Can you work these out from the model? Positions are in its coordinate system, mm. A direction names the side the tool comes from. Coordinates: 2 decimals unless noted, no trailing zeros. Order: outer loops, then holes, each group sorted by start corner. A loop starts at its lowest first (then second) coordinate and runs counter-clockwise, first axis right, second up.
```python
from build123d import *

# Parameters (mm, degrees)
SKETCH1_W           = 30
SKETCH1_H           = 52
SKETCH1_R           = 1.9
BOSS_EXTRUDE1_DEPTH = 10
CHAMFER1_SIZE       = 15
CHAMFER1_SIZE2      = 2.644904711
SKETCH2_W           = 5
SKETCH2_H           = 7.355095289
SKETCH2_H_2         = 30
BOSS_EXTRUDE2_DEPTH = 10
SKETCH3_R           = 1
SKETCH3_R_2         = 1.5
SKETCH3_R_3         = 2
CUT_EXTRUDE1_DEPTH  = 35
CHAMFER2_SIZE       = 1


with BuildPart() as part:
    # Sketch1 → Boss-Extrude1 (new body)
    with BuildSketch(Plane.XY):
        with Locations((15, 6)):
            Rectangle(SKETCH1_W, SKETCH1_H)
        with Locations((4.5, 26.5)):
            Circle(SKETCH1_R, mode=Mode.SUBTRACT)
        with Locations((25.5, 26.5)):
            Circle(SKETCH1_R, mode=Mode.SUBTRACT)
        with Locations((25.5, 5.5)):
            Circle(SKETCH1_R, mode=Mode.SUBTRACT)
        with Locations((4.5, 5.5)):
            Circle(SKETCH1_R, mode=Mode.SUBTRACT)
    extrude(amount=BOSS_EXTRUDE1_DEPTH)

    # Chamfer1
    chamfer1_edges = [part.edges().sort_by_distance(p)[0] for p in [
        (15, -20, 0),
    ]]
    chamfer1_side = [part.faces().sort_by_distance(p)[0] for p in [
        (15, 5.700491631, 0),
    ]]
    chamfer(chamfer1_edges, length=CHAMFER1_SIZE, length2=CHAMFER1_SIZE2, reference=chamfer1_side[0])

    # Sketch2 → Boss-Extrude2 (add)
    with BuildSketch(Plane.XZ.offset(20)):
        Polygon((0, 10), (30, 10), (30, 50), (-55, 50), (-55, 20), (-55, 10), (-5, 10), align=None)
        Polygon((-5, 2.644904711), (-5, 10), (-55, 10), (-55, -30), (-5, -30), align=None)
        with Locations((-2.5, 6.322452356)):
            Rectangle(SKETCH2_W, SKETCH2_H)
        with Locations((-57.5, 35)):
            Rectangle(SKETCH2_W, SKETCH2_H_2)
    extrude(amount=-BOSS_EXTRUDE2_DEPTH)

    # Sketch3 → Cut-Extrude1 (cut)
    with BuildSketch(Plane(origin=(0, -10, 0), x_dir=(1, 0, 0), z_dir=(0, 1, 0))):
        with Locations(Location((-43.5, 8, 0), (0, 0, 270))):
            Circle(SKETCH3_R)
        with Locations(Location((-43.5, 3, 0), (0, 0, 270))):
            Circle(SKETCH3_R_2)
        with Locations(Location((-33.5, -33.25, 0), (0, 0, 270))):
            Circle(SKETCH3_R_3)
        with Locations(Location((-53.5, -33.25, 0), (0, 0, 270))):
            Circle(SKETCH3_R_3)
        with Locations(Location((-43.5, -33.25, 0), (0, 0, 270))):
            Circle(SKETCH3_R_3)
    extrude(amount=-CUT_EXTRUDE1_DEPTH, mode=Mode.SUBTRACT)

    # Chamfer2
    chamfer2_edges = [part.edges().sort_by_distance(p)[0] for p in [
        (0, 32, 5),
        (30, 32, 5),
        (-15, -10, 50),
        (30, -15, 50),
        (-30, -10, -30),
        (-5, -15, -30),
        (-55, -15, -30),
        (-55, -20, -5),
        (-15, -20, 50),
        (-30, -20, -30),
        (-55, -10, -5),
        (15, -10, 10),
        (0, -10, 6.322452355),
    ]]
    chamfer(chamfer2_edges, length=CHAMFER2_SIZE)


solid = part.part
```
1. Imagine slicing it at A-A on x = 4.5. Please give me the cut outline in (y, z), then the cut area to 3 significant figures.
Completed:
outline: (-20, 2.64) - (-5, 0) - (3.6, 0) - (3.6, 10) - (-9, 10) - (-10, 11) - (-10, 49) - (-11, 50) - (-19, 50) - (-20, 49) - close; (7.4, 0) - (24.6, 0) - (24.6, 10) - (7.4, 10) - close; (28.4, 0) - (32, 0) - (32, 10) - (28.4, 10) - close
area: 824 mm2
2. I'm going to push flat-ended pins straight in: pin 1 (5 mm diameter, centred on x = -28, z = -17, fed in from +Y); pin 2 (6.5 mm diameter, centred on x = -58, y = -15.5, fed in from -Z); pin 3 (12 mm diameter, centred on y = 4, z = 15.5, fed in from -X). Where does each tip first touch, or does it pass through?
Completed:
pin 1: stops at y = -10
pin 2: stops at z = -29.25
pin 3: stops at x = 0
3. On a 3-axis mill with a long thin cutter (end or side, diameter ignored), from which of +Z, -Z, +X, -X, +Y, -Y can I reach the whole of each face in a straight line? I mean faces 1 (the cylindrical face through (-35.274, -14.93, 34.173)), 2 (the flat face through (15, 12, 10)), 3 (the flat face through (-3, -15, 2.645)). Say none if no direction works.
Completed:
face 1: +Y, -Y
face 2: +Z, +X, -X, +Y
face 3: -Z, +Y, -Y
4. Imagine slicing it at C-C on x = -33.5. Please give me the cut outline in (y, z), then the cut area to 3 significant figures.
Completed:
outline: (-20, -29) - (-19, -30) - (-11, -30) - (-10, -29) - (-10, 31.25) - (-20, 31.25) - close; (-20, 35.25) - (-10, 35.25) - (-10, 49) - (-11, 50) - (-19, 50) - (-20, 49) - close
area: 758 mm2
5. Imagine slicing it at D-D on x = 22. Please give me the cut outline in (y, z), then the cut area to 3 significant figures.
Completed:
outline: (-20, 2.64) - (-5, 0) - (32, 0) - (32, 10) - (-9, 10) - (-10, 11) - (-10, 49) - (-11, 50) - (-19, 50) - (-20, 49) - close
area: 900 mm2
6. Thinking about a two-plate mould opening in Y: for faces 4 (the flat face through (14.79, -12.6, 1.34)), 5 (the flat face through (-55, -15, -4)), 6 (the cylindrical face through (4.253, 28.384, 4.93)), which applies, pulls with the +Y half, pulls with the -Y half, needs draft (parallel to the pull), parting line crosses it, or undercut?
Completed:
face 4: pulls with the -Y half
face 5: needs draft
face 6: undercut
7. Please list where these lines run through material, in increasing order: probe 1 along Y at (x, z) = (25.5, 3); probe 2 along X at (y, z) = (5, 3); probe 3 along X at (y, z) = (-17, 33).
Completed:
probe 1: y = -20 to 3.6, 7.4 to 24.6, 28.4 to 32
probe 2: x = 0 to 2.67, 6.33 to 23.67, 27.33 to 30
probe 3: x = -60 to -55.48, -51.52 to -45.48, -41.52 to -35.48, -31.52 to 30
8. Imagine slicing it at B-B on z = 33.25. Please give me the cut outline in (x, y), then the cut area to 3 significant figures.
Completed:
outline: (-60, -20) - (-55.5, -20) - (-55.5, -10) - (-60, -10) - close; (-51.5, -20) - (-45.5, -20) - (-45.5, -10) - (-51.5, -10) - close; (-41.5, -20) - (-35.5, -20) - (-35.5, -10) - (-41.5, -10) - close; (-31.5, -20) - (30, -20) - (30, -10) - (-31.5, -10) - close
area: 780 mm2
